For this review, take the finished solid that the model builds, in its own axes (mm). Face numbers are marked on the shaded views. Give positions to 0.01 mm unless a question says otherwise; leave off trailing zeros. Order: outer loops, then holes, each group sorted by start corner. A loop starts at its lowest first (then second) coordinate and runs counter-clockwise, first axis right, second up.
Item 1: Consider section C-C (y = 3.5). Give the boundary of the cut face in (x, z).
Item 2: For probe 1 along Z at (x, y) = (-21, 0); probe 2 along Y at (x, z) = (0, -42) (3 decimals); probe 3 along Y at (x, z) = (-21.05, -45), list the stretches that pass through material, from the lowest coordinate up.
Item 3: Consider section B-B (x = 0). Give the boundary of the cut face in (y, z) (3 decimals).
Item 4: Consider section D-D (z = -53.5). Give the boundary of the cut face in (x, y) (3 decimals).
Item 5: The part is to be moulded in two halves that separate along Y. For the marked faces 1, 2, 3 and 4, say which applies: released by +Y, released by -Y, zero draft, split by the parting line, or undercut.
Item 6: Consider section A-A (z = -45). Give the boundary of the cut face in (x, y) (3 decimals).
Item 7: For P1, Ø3.5, axis at y = 0, z = -45, coming from the +X side, flat-tipped, find the tip position at first contact; note if it passes through.
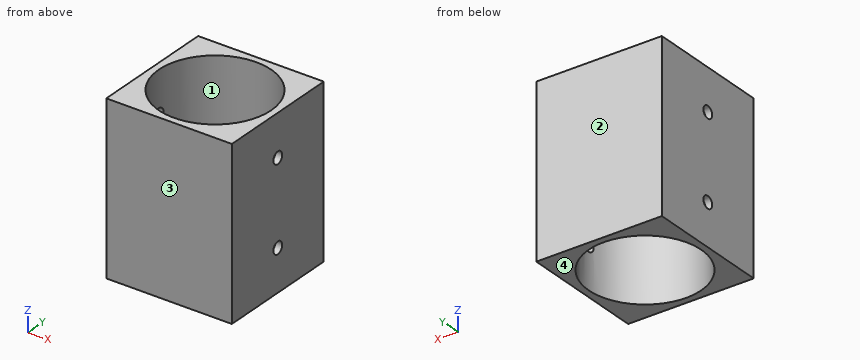
Autodesk Inventor part; units mm, degrees
ref_plane "YZ Plane" through (0, 0, 0) normal (1, 0, 0) x (0, 1, 0)
ref_plane "XZ Plane" through (0, 0, 0) normal (0, 1, 0) x (-1, 0, 0)
ref_plane "XY Plane" through (0, 0, 0) normal (0, 0, 1) x (1, 0, 0)
sketch "Sketch1" plane through (0, 0, 0) normal (1, 0, 0) x (0, 1, 0)
  line L0 (0, 0) -> (0, -15)
  line L1 (0, -15) -> (0, -45)
  line L2 (0, -45) -> (0, -60)
  dimension "d0" = 15
  dimension "d2" = 30
  dimension "d3" = 15
sketch "Sketch2" plane through (0, 0, 0) normal (0, 0, 1) x (1, 0, 0)
  line L0 (-22.5, 22.5) -> (22.5, 22.5)
  line L1 (22.5, 22.5) -> (22.5, -22.5)
  line L2 (22.5, -22.5) -> (-22.5, -22.5)
  line L3 (-22.5, -22.5) -> (-22.5, 22.5)
  line L4 (-22.5, 22.5) -> (22.5, -22.5) construction
  line L5 (22.5, 22.5) -> (-22.5, -22.5) construction
  circle A0 centre (0, 0) radius 20.125
  dimension "d6" = 45
  dimension "d7" = 45
  dimension "d8" = 40.25
extrude "Extrusion1" add sketch "Sketch2" against normal blind 60
hole "Hole1" at (0, 0, -15) at (0, 0, -45) direction (-1, 0, 0) diameter 4.3 end through all both
properties part number "Bohrschablone_Oben"
Resolved:
1. outline: (-22.5, -60) - (-19.82, -60) - (-19.82, 0) - (-22.5, 0) - close; (19.82, -60) - (22.5, -60) - (22.5, 0) - (19.82, 0) - close
2. probe 1: z = -60 to -47.15, -42.85 to -17.15, -12.85 to 0
2. probe 2: y = -22.5 to -20.125, 20.125 to 22.5
2. probe 3: y = -22.5 to -2.15, 2.15 to 22.5
3. outline: (-22.5, -60) - (-20.125, -60) - (-20.125, 0) - (-22.5, 0) - close; (20.125, -60) - (22.5, -60) - (22.5, 0) - (20.125, 0) - close
4. outline: (-22.5, -22.5) - (22.5, -22.5) - (22.5, 22.5) - (-22.5, 22.5) - close; hole circle Ø40.25 at (0, 0)
5. face 1: undercut
5. face 2: released by +Y
5. face 3: released by -Y
5. face 4: zero draft
6. outline: (-22.5, -22.5) - (22.5, -22.5) - (22.5, -2.15) - (20.01, -2.15) arc R20.125 cw to (-20.01, -2.15) - (-22.5, -2.15) - close; (-22.5, 2.15) - (-20.01, 2.15) arc R20.125 cw to (20.01, 2.15) - (22.5, 2.15) - (22.5, 22.5) - (-22.5, 22.5) - close
7. P1: passes through
